```python
from build123d import *

# Parameters (mm, degrees)
SKETCH1_R           = 4.09575
SKETCH1_R_2         = 1.651
BOSS_EXTRUDE1_DEPTH = 6.35
SKETCH3_R           = 1.5875
CUT_EXTRUDE1_DEPTH  = 6.35
CUT_EXTRUDE2_DEPTH  = 6.35
SKETCH7_R           = 4.9784
CUT_EXTRUDE3_DEPTH  = 125.084268237
FILLET1_R           = 6.35
SKETCH8_W           = 50.8
SKETCH8_H           = 12.7
CUT_EXTRUDE4_DEPTH  = 50.8
CUT_EXTRUDE5_DEPTH  = 19.304
FILLET6_R           = 6.35
FILLET7_R           = 6.35
FILLET8_R           = 19.05
SKETCH10_R          = 1.5875
CUT_EXTRUDE6_DEPTH  = 6.35
SKETCH11_R          = 1.5875
CUT_EXTRUDE7_DEPTH  = 6.35
BOSS_EXTRUDE2_DEPTH = 6.35
FILLET9_R           = 24.13


with BuildPart() as part:
    # Sketch1 → Boss-Extrude1 (new body)
    with BuildSketch(Plane.XY):
        with BuildLine():
            Line((0, 0), (107.95, 0))
            Line((107.95, 0), (100.9362606, 26.175631792))
            Line((100.9362606, 26.175631792), (100.868755024, 26.427566033))
            ThreePointArc((100.868755024, 26.427566033), (110.348359368, 43.438223217), (95.367453293, 55.88))
            Line((95.367453293, 55.88), (0, 38.1))
            Line((0, 38.1), (0, 25.4))
            Line((0, 25.4), (-7.62, 25.4))
            Line((-7.62, 25.4), (-7.62, 12.7))
            Line((-7.62, 12.7), (0, 12.7))
            Line((0, 12.7), (0, 0))
        make_face()
        with Locations((95.367453293, 40.64)):
            Circle(SKETCH1_R, mode=Mode.SUBTRACT)
        with Locations((25.817011896, 25.817011896)):
            Circle(SKETCH1_R_2, mode=Mode.SUBTRACT)
        with Locations((25.817011896, 12.282988104)):
            Circle(SKETCH1_R_2, mode=Mode.SUBTRACT)
        with Locations((12.282988104, 12.282988104)):
            Circle(SKETCH1_R_2, mode=Mode.SUBTRACT)
        with Locations((12.282988104, 25.817011896)):
            Circle(SKETCH1_R_2, mode=Mode.SUBTRACT)
    extrude(amount=BOSS_EXTRUDE1_DEPTH)

    # Sketch3 → Cut-Extrude1 (cut)
    with BuildSketch(Plane.ZY):
        with Locations(Location((3.175, 31.75, 0), (0, 0, 270))):
            Circle(SKETCH3_R)
        with Locations(Location((3.175, 6.35, 0), (0, 0, 270))):
            Circle(SKETCH3_R)
    extrude(amount=-CUT_EXTRUDE1_DEPTH, mode=Mode.SUBTRACT)

    # Sketch6 → Cut-Extrude2 (cut)
    with BuildSketch(Plane.XY.offset(6.35)):
        with BuildLine():
            Line((50.8, 0), (76.2, 0))
            ThreePointArc((76.2, 0), (63.5, 12.7), (50.8, 0))
        make_face()
    extrude(amount=-CUT_EXTRUDE2_DEPTH, mode=Mode.SUBTRACT)

    # Sketch7 → Cut-Extrude3 (cut, through all)
    with BuildSketch(Plane.XY.offset(6.35)):
        with Locations((19.05, 19.05)):
            Circle(SKETCH7_R)
    extrude(amount=-CUT_EXTRUDE3_DEPTH, mode=Mode.SUBTRACT)

    # Fillet1
    fillet1_edges = [part.edges().sort_by_distance(p)[0] for p in [
        (100.868755024, 26.427566033, 3.175),
    ]]
    fillet(fillet1_edges, radius=FILLET1_R)

    # Sketch8 → Cut-Extrude4 (cut)
    with BuildSketch(Plane.XY.offset(6.35)):
        with Locations((25.4, 44.45)):
            Rectangle(SKETCH8_W, SKETCH8_H)
    extrude(amount=-CUT_EXTRUDE4_DEPTH, mode=Mode.SUBTRACT)

    # Sketch9 → Cut-Extrude5 (cut)
    with BuildSketch(Plane.XY.offset(6.35)):
        Polygon((50.8, 47.57098794), (50.8, 40.64), (57.15, 40.64), (57.15, 48.754861432), align=None)
    extrude(amount=-CUT_EXTRUDE5_DEPTH, mode=Mode.SUBTRACT)

    # Fillet6
    fillet6_edges = [part.edges().sort_by_distance(p)[0] for p in [
        (57.15, 40.64, 3.175),
    ]]
    fillet(fillet6_edges, radius=FILLET6_R - 0.0001)  # a hair under: the kernel refuses the full size

    # Fillet7
    fillet7_edges = [part.edges().sort_by_distance(p)[0] for p in [
        (57.15, 48.754861432, 3.175),
    ]]
    fillet(fillet7_edges, radius=FILLET7_R)

    # Fillet8
    fillet8_edges = [part.edges().sort_by_distance(p)[0] for p in [
        (50.8, 0, 3.175),
    ]]
    fillet(fillet8_edges, radius=FILLET8_R)

    # Sketch10 → Cut-Extrude6 (cut)
    with BuildSketch(Plane.XZ):
        with Locations(Location((97.79, 3.175, 0), (0, 0, 270))):
            Circle(SKETCH10_R)
        with Locations(Location((86.36, 3.175, 0), (0, 0, 270))):
            Circle(SKETCH10_R)
        with Locations(Location((31.75, 3.175, 0), (0, 0, 270))):
            Circle(SKETCH10_R)
        with Locations(Location((12.7, 3.175, 0), (0, 0, 270))):
            Circle(SKETCH10_R)
    extrude(amount=-CUT_EXTRUDE6_DEPTH, mode=Mode.SUBTRACT)

    # Sketch11 → Cut-Extrude7 (cut)
    with BuildSketch(Plane(origin=(0, 38.1, 0), x_dir=(1, 0, 0), z_dir=(0, 1, 0))):
        with Locations(Location((12.7, -2.922371253, 0), (0, 0, 270))):
            Circle(SKETCH11_R)
        with Locations(Location((25.4, -2.922371253, 0), (0, 0, 270))):
            Circle(SKETCH11_R)
        with Locations(Location((38.1, -2.922371253, 0), (0, 0, 270))):
            Circle(SKETCH11_R)
    extrude(amount=-CUT_EXTRUDE7_DEPTH, mode=Mode.SUBTRACT)

    # Sketch12 → Boss-Extrude2 (add)
    with BuildSketch(Plane.XY.offset(6.35)):
        with BuildLine():
            Line((50.8, 40.64), (85.027112904, 40.64))
            Line((85.027112904, 40.64), (95.367453293, 55.88))
            add(Edge.make_bspline(
                [(50.8, 40.64), (70.777788932, 52.178803671), (78.594281742, 111.543427795), (95.367453293, 55.88)],
                knots=[0, 0, 0, 0, 1, 1, 1, 1], degree=3))
        make_face()
    extrude(amount=-BOSS_EXTRUDE2_DEPTH)

    # Fillet9
    fillet9_edges = [part.edges().sort_by_distance(p)[0] for p in [
        (95.367453293, 55.88, 3.175),
    ]]
    fillet(fillet9_edges, radius=FILLET9_R)


solid = part.part
```
Here's how the part is built. I have some questions about the finished solid (model axes, mm). A direction names the side the tool comes from. Coordinates: 2 decimals unless noted, no trailing zeros. Write each loop counter-clockwise with the first axis right and the second up, starting at its lowest first coordinate (ties: lowest second). Pieces come first, ordered by that corner, then holes. Notation, with made-up numbers: M 31.25,62 L 51.25,62 A21 ccw 51.25,86 Z; hole C 38,8.5 d11. An arc over 180 degrees is marked long. Answer as CSV lines item,"result". Start each with the question number.
Q1. Will these pins go through, and if not, where does the flat tip stop? pin 1 Ø3 at (y, z) = (30, 1.5) entering from -X; pin 2 Ø3 at (x, z) = (25.4, 2.92) entering from +Y; pin 3 Ø4.5 at (x, y) = (12.28, 12.28) entering from -Z; pin 4 Ø3.5 at (x, z) = (12.5, 2.5) entering from +Y.
Q2. Suppose I cut it at B-B, the plane x = 31.75. List the corners of the cut face in (y, z) for me.
Q3. If we mould it in two halves opening along Y, with no side actions, what happens to faces 1 (the cylindrical face through (3.131, 5.497, 4.514)), 2 (the cylindrical face through (87.934, 3.131, 3.382)), 3 (the flat face through (32, 6.35, 3))? For each: pulls with the +Y half, pulls with the -Y half, needs draft (parallel to the pull), parting line crosses it, or undercut.
Q4. Suppose I cut it at A-A, the plane x = 19.05. List the corners of the cut face in (y, z) for me.
Q5. I need wall thicknesses on probe 1 along Z at (x, y) = (3.25, 6.35); probe 2 along Y at (x, z) = (3.5, 3); probe 3 along Y at (x, z) = (27, 4). Which ranges of each line are inside material? Lowest first, please. Write a range as [from, to].
Q6. For faces 4 (the flat face through (86, 6.35, 3)), 5 (the flat face through (105.085, 10.692, 3.131)), 6 (the flat face through (25, 38.1, 5)), 7 (the flat face through (38, 31.75, 3)), 8 (the flat face through (-4, 12.7, 3)), which set-ups out of +Z, -Z, +X, -X, +Y, -Y let a thin tool reach every point of the face, with its end or its side?
Entries:
1,pin 1,"stops at x = 0"
1,pin 2,"stops at y = 31.75"
1,pin 3,"stops at z = 0"
1,pin 4,"stops at y = 38.1"
2,outline,"M 0,0 L 38.1,0 L 38.1,6.35 L 0,6.35 L 0,4.76 L 6.35,4.76 L 6.35,1.59 L 0,1.59 Z"
3,face 1,"undercut"
3,face 2,"needs draft"
3,face 3,"pulls with the -Y half"
4,outline,"M 0,0 L 14.07,0 L 14.07,6.35 L 0,6.35 Z; M 24.03,0 L 38.1,0 L 38.1,6.35 L 24.03,6.35 Z"
5,probe 1,"z = [0, 1.59], [4.76, 6.35]"
5,probe 2,"y = [0, 4.77], [7.93, 30.17], [33.33, 38.1]"
5,probe 3,"y = [0, 11.13], [13.43, 24.67], [26.97, 38.1]"
6,face 4,"-Y"
6,face 5,"+Z, -Z, +X"
6,face 6,"+Z, -Z, -X, +Y"
6,face 7,"+Y"
6,face 8,"+Z, -Z, -X, -Y"
